```python
from build123d import *

# Parameters (mm, degrees)
EXTRUDE_1_DEPTH      = 12
CUT_EXTRUDE_1_DEPTH  = 52.946106026
CUT_EXTRUDE_2_DEPTH  = 52.946106026
CUT_EXTRUDE_3_DEPTH  = 51.68530359
EXTRUDE_2_DEPTH      = 7
EXTRUDE_2_DEPTH_BACK = 7
SKETCH_6_W           = 8
SKETCH_6_H           = 2
CUT_EXTRUDE_4_DEPTH  = 5
SKETCH_7_W           = 4
SKETCH_7_H           = 8
CUT_EXTRUDE_5_DEPTH  = 5
SKETCH_8_W           = 5
SKETCH_8_H           = 5
CUT_EXTRUDE_6_DEPTH  = 2


with BuildPart() as part:
    # Эскиз1 → Бобышка-Вытянуть1 (new body)
    with BuildSketch(Plane.XY):
        Polygon((-10, 45), (10, 45), (20, 0), (-20, 0), align=None)
    extrude(amount=EXTRUDE_1_DEPTH)

    # Эскиз2 → Вырез-Вытянуть1 (cut, through all, along a direction that is not the sketch's normal)
    with BuildSketch(Plane.XZ):
        Polygon((-20, 0), (-20, 12), (-17, 12), align=None)
    extrude(amount=-CUT_EXTRUDE_1_DEPTH, dir=(-0.21693045781865616, -0.9761870601839528, 0), mode=Mode.SUBTRACT)

    # Эскиз3 → Вырез-Вытянуть2 (cut, through all, along a direction that is not the sketch's normal)
    with BuildSketch(Plane.XZ):
        Polygon((20, 0), (20, 12), (17, 12), align=None)
    extrude(amount=-CUT_EXTRUDE_2_DEPTH, dir=(0.21693045781865616, -0.9761870601839528, 0), mode=Mode.SUBTRACT)

    # Эскиз4 → Вырез-Вытянуть3 (cut, through all)
    with BuildSketch(Plane(origin=(0, 45, 0), x_dir=(1, 0, 0), z_dir=(0, 1, 0))):
        Polygon((0, 0), (-2.5, 0), (0, -4), (2.5, 0), align=None)
    extrude(amount=-CUT_EXTRUDE_3_DEPTH, mode=Mode.SUBTRACT)

    # Эскиз5 → Бобышка-Вытянуть2 (add, two sides: drawn at the far end of the back side and taken through both)
    with BuildSketch(Plane(origin=(0, 0, 0), x_dir=(0, 0, -1), z_dir=(1, 0, 0)).offset(-EXTRUDE_2_DEPTH_BACK)):
        Polygon((-12, 0), (-32, 0), (-32, 35), (-28, 35), (-28, 13), (-12, 13), align=None)
    extrude(amount=EXTRUDE_2_DEPTH + EXTRUDE_2_DEPTH_BACK)

    # Эскиз6 → Вырез-Вытянуть4 (cut)
    with BuildSketch(Plane.XY.offset(32)):
        with Locations((0, 1)):
            Rectangle(SKETCH_6_W, SKETCH_6_H)
    extrude(amount=-CUT_EXTRUDE_4_DEPTH, mode=Mode.SUBTRACT)

    # Эскиз7 → Вырез-Вытянуть5 (cut)
    with BuildSketch(Plane.ZY.offset(7)):
        with Locations((30, 28)):
            Rectangle(SKETCH_7_W, SKETCH_7_H)
    extrude(amount=-CUT_EXTRUDE_5_DEPTH, mode=Mode.SUBTRACT)

    # Эскиз8 → Вырез-Вытянуть6 (cut)
    with BuildSketch(Plane(origin=(-7, 0, 0), x_dir=(0, 0, -1), z_dir=(1, 0, 0))):
        with Locations((-25.5, 6.5)):
            Rectangle(SKETCH_8_W, SKETCH_8_H)
    extrude(amount=CUT_EXTRUDE_6_DEPTH, mode=Mode.SUBTRACT)


solid = part.part
```
Check sheet for the modelled part. Datum: model origin and axes. Units: mm. A direction names the side the tool comes from. Give positions to 0.01 mm unless a question says otherwise; leave off trailing zeros. Order: outer loops, then holes, each group sorted by start corner. A loop starts at its lowest first (then second) coordinate and runs counter-clockwise, first axis right, second up. Notation, with made-up numbers: (68.5, 82.5) -> (74.5, 82.5) arc R15 ccw to (74.5, 98.5) -> close; hole circle Ø1 at (51.25, 32.25). An arc over 180 degrees is marked (long way). Return JSON: item names as keys, results as strings.
1. Cross-section at D-D, the plane z = 3. Record the cut outline in (x, y) (3 decimals).
From the geometry:
{"outline": "(-19.25, 0) -> (-0.625, 0) -> (-0.625, 45) -> (-9.25, 45) -> close; (0.625, 0) -> (19.25, 0) -> (9.25, 45) -> (0.625, 45) -> close"}
2. Cross-section at B-B, the plane z = 24. Record the cut outline in (x, y).
From the geometry:
{"outline": "(-7, 0) -> (7, 0) -> (7, 13) -> (-7, 13) -> (-7, 9) -> (-5, 9) -> (-5, 4) -> (-7, 4) -> close"}
3. Material ranges on probe 1 along Y at (x, z) = (-4.5, 22); probe 2 along X at (y, z) = (2, 12.5); probe 3 along Z at (x, y) = (5, 31.5), recorded low to high. Write a range as [from, to].
From the geometry:
{"probe 1": "[0, 13]", "probe 2": "[-7, 7]", "probe 3": "[0, 12], [28, 32]"}
4. Go/stop test with flat-tipped pins: P1, Ø1.5, axis at y = 33, z = 30.5, coming from the -X side; P2, Ø2, axis at y = 5.5, z = 11, coming from the -X side; P3, Ø0.6, axis at x = 2, y = 1, coming from the +Z side. Record where each tip stops, or that it passes through.
From the geometry:
{"P1": "x = -7", "P2": "x = -16.36", "P3": "z = 27"}
5. Mould release check, pull along X, two halves, no side actions. Record for faces 6 (the flat face through (-6, 4, 26)), 7 (the flat face through (-1.27, 22.82, 1.97)), 8 (the flat face through (-13.54, 22.18, 6.12)): +X half, -X half, draft (parallel to the pull), parting line (faces both ways), or undercut.
From the geometry:
{"face 6": "draft", "face 7": "undercut", "face 8": "-X half"}
6. Cross-section at A-A, the plane y = 14.5. Record the cut outline in (x, z).
From the geometry:
{"outline": "(-16.78, 0) -> (-2.5, 0) -> (0, 4) -> (2.5, 0) -> (16.78, 0) -> (13.78, 12) -> (-13.78, 12) -> close; (-7, 28) -> (7, 28) -> (7, 32) -> (-7, 32) -> close"}
7. Set-up check for faces 1 (the flat face through (-7, 10, 22)), 2 (the flat face through (1, 24, 28)), 3 (the flat face through (0, 23, 12)), 4 (the flat face through (0, 2, 30)), 5 (the flat face through (-6, 6, 23)): record each of +Z, -Z, +X, -X, +Y, -Y from which the full face is reachable in a straight line by a thin tool's end or side.
From the geometry:
{"face 1": "+Z, -X, +Y, -Y", "face 2": "+X, -X, +Y", "face 3": "+Y", "face 4": "+Z, -Y", "face 5": "-X"}
8. Cross-section at C-C, the plane x = 14.5. Record the cut outline in (y, z).
From the geometry:
{"outline": "(0, 0) -> (24.75, 0) -> (11.25, 12) -> (0, 12) -> close"}
